Check sheet for the modelled part. Datum: model origin and axes. Units: mm. A direction names the side the tool comes from. Give positions to 0.01 mm unless a question says otherwise; leave off trailing zeros. Order: outer loops, then holes, each group sorted by start corner. A loop starts at its lowest first (then second) coordinate and runs counter-clockwise, first axis right, second up.
from build123d import *

# Parameters (mm, degrees)
F1_DEPTH = 15


with BuildPart() as f1:
    # F0 (on Top) → F1 (new body)
    with BuildSketch(Plane.XY):
        Polygon((0, 200), (0, 0), (575, 0), (575, 40), (685, 40), (685, 80), (565, 123.676428), (565, 1109.50136), (685, 1120), (685, 1160), (0, 1160), (0, 960), (-60, 960), (-60, 860), (0, 860), (0, 300), (-60, 300), (-60, 200), align=None)
    extrude(amount=F1_DEPTH)


solid = f1.part
1) Section check C-C, the plane y = 344. Record the cut outline in (x, z).
Recorded:
outline: (0, 0) - (565, 0) - (565, 15) - (0, 15) - close
2) Material ranges on L1, parallel to X at y = 548.5, z = 14; L2, parallel to X at y = 297, z = 14, recorded low to high.
Recorded:
L1: x = 0 to 565
L2: x = -60 to 565
3) Section check A-A, the plane x = 614.5. Record the cut outline in (y, z).
Recorded:
outline: (40, 0) - (105.66, 0) - (105.66, 15) - (40, 15) - close; (1113.83, 0) - (1160, 0) - (1160, 15) - (1113.83, 15) - close
4) Depth check by flat-ended pin: pin 1 Ø4.5 at (x, z) = (-33.5, 4) entering from -Y; pin 2 Ø4.5 at (y, z) = (144.5, 5.5) entering from -X; pin 3 Ø4.5 at (x, z) = (654, 5) entering from -Y. Enter the tip coordinate at first touch or a pass-through.
Recorded:
pin 1: stops at y = 200
pin 2: stops at x = 0
pin 3: stops at y = 40
5) Set-up check for faces 1 (the face through (625.84, 101.532, 7.395)), 2 (the face through (307, 588, 15)): record each of +Z, -Z, +X, -X, +Y, -Y from which the full face is reachable in a straight line by a thin tool's end or side.
Recorded:
face 1: +Z, -Z, +X
face 2: +Z, +X, -X, +Y, -Y
6) Section check B-B, the plane z = 7.75. Record the cut outline in (x, y), then the cut area to 3 significant figures.
Recorded:
outline: (-60, 200) - (0, 200) - (0, 0) - (575, 0) - (575, 40) - (685, 40) - (685, 80) - (565, 123.68) - (565, 1109.5) - (685, 1120) - (685, 1160) - (0, 1160) - (0, 960) - (-60, 960) - (-60, 860) - (0, 860) - (0, 300) - (-60, 300) - close
area: 681,000 mm2
